Verification items for the finished model (mm, model axes). Face numbers are marked on the shaded views. A direction names the side the tool comes from. Round coordinates to 2 decimals unless told otherwise and drop trailing zeros. Loops run counter-clockwise (first coordinate to the right, second up) from the corner with the lowest first, then second, coordinate; pieces in that order, holes last. Notation, with made-up numbers: (61.25, 22) - (112.25, 22) arc R28 ccw to (112.25, 53) - close; hole circle Ø3 at (50, 74.5). An arc over 180 degrees is marked (long way). Use a Markdown table: item, result. Add a question column.
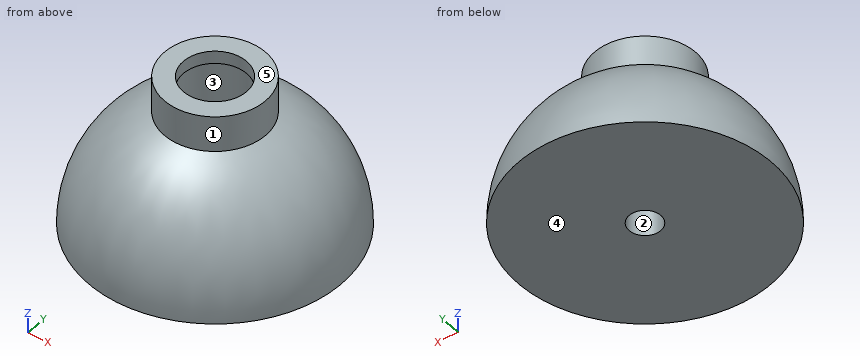
```python
from build123d import *

# Parameters (mm, degrees)
F1_R     = 25.4
F1_R_2   = 10.16
F2_DEPTH = 25.4
F3_R     = 25.39999
F4_DEPTH = 30.48
F7_D     = 16.51
F8_DEPTH = 7.62
F9_START = 27.94
F9_DEPTH = 2.54


# Not quite as in the source:
# - a variable given as a bare number and used for a length is read in inches; the dataset says mm whatever the document's units were
# - a fillet or chamfer is up to 0.001 mm smaller than in the source, because OpenCascade refuses the exact size


with BuildPart() as f2:
    # F1 (on Top) → F2 (new body)
    with BuildSketch(Plane.XY):
        Circle(F1_R)
        Circle(F1_R_2, mode=Mode.SUBTRACT)
        Circle(F1_R_2)
    extrude(amount=F2_DEPTH)

    # F3 (radius 25.4 in the source; OpenCascade refuses exactly that, so slightly less here)
    f3_edges = [f2.edges().sort_by_distance(p)[0] for p in [
        (-25.4, 0, 25.4),
    ]]
    fillet(f3_edges, radius=F3_R)

    # F1 (on Top) → F4 (join)
    with BuildSketch(Plane.XY):
        Circle(F1_R_2)
    extrude(amount=F4_DEPTH)

    # F7 (through all)
    with Locations(Plane(origin=(0, 0, 0), x_dir=(1, 0, 0), z_dir=(0, 0, -1))):
        with Locations((0, 0)):
            Hole(F7_D / 2)

    # F6 (on face) → F8 (join)
    with BuildSketch(Plane.XY):
        with BuildLine():
            ThreePointArc((-6.35, 0), (0, -6.35), (6.35, 0))
            Line((6.35, 0), (3.175, 0))
            ThreePointArc((3.175, 0), (0, -3.175), (-3.175, 0))
            Line((-3.175, 0), (-6.35, 0))
        make_face()
        with BuildLine():
            Line((3.175, 0), (6.35, 0))
            ThreePointArc((6.35, 0), (0, 6.35), (-6.35, 0))
            Line((-6.35, 0), (-3.175, 0))
            ThreePointArc((-3.175, 0), (0, 3.175), (3.175, 0))
        make_face()
        with BuildLine():
            Line((8.255, 0), (6.35, 0))
            ThreePointArc((6.35, 0), (0, -6.35), (-6.35, 0))
            Line((-6.35, 0), (-8.255, 0))
            ThreePointArc((-8.255, 0), (0, -8.255), (8.255, 0))
        make_face()
        with BuildLine():
            ThreePointArc((-6.35, 0), (0, 6.35), (6.35, 0))
            Line((6.35, 0), (8.255, 0))
            ThreePointArc((8.255, 0), (0, 8.255), (-8.255, 0))
            Line((-8.255, 0), (-6.35, 0))
        make_face()
    extrude(amount=F8_DEPTH)

    # F6 (on face) → F9 (join)
    with BuildSketch(Plane.XY.offset(F9_START)):
        with BuildLine():
            Line((8.255, 0), (6.35, 0))
            ThreePointArc((6.35, 0), (0, -6.35), (-6.35, 0))
            Line((-6.35, 0), (-8.255, 0))
            ThreePointArc((-8.255, 0), (0, -8.255), (8.255, 0))
        make_face()
        with BuildLine():
            ThreePointArc((-6.35, 0), (0, 6.35), (6.35, 0))
            Line((6.35, 0), (8.255, 0))
            ThreePointArc((8.255, 0), (0, 8.255), (-8.255, 0))
            Line((-8.255, 0), (-6.35, 0))
        make_face()
    extrude(amount=F9_DEPTH)


solid = f2.part
```
Q1. Release check for a two-part mould opening along Z. For the marked faces 3, 4 and 5 record: +Z half, -Z half, draft (parallel to the pull), parting line (faces both ways), or undercut.
Q2. Go/stop test with flat-tipped pins: pin 1 Ø10 at (x, z) = (-14, 23.5) entering from -Y; pin 2 Ø4 at (x, z) = (-1, 13) entering from +Y; pin 3 Ø4 at (x, z) = (-6.5, 7) entering from -Y. Record where each tip stops, or that it passes through.
Q3. Section check A-A on z = 25.5. Record the cut outline in (x, y) (3 decimals).
Q4. Set-up check for the marked faces 1 and 2: record each of +Z, -Z, +X, -X, +Y, -Y from which the full face is reachable in a straight line by a thin tool's end or side.
Q5. Thickness scan on line 1 along Y through (x, z) = (0, 28.95); line 2 along Z through (x, y) = (-7.5, 1.5); line 3 along Y through (x, z) = (0, 5) (3 decimals). Record the ranges inside material, lowest first.
Determined:
| question | item | result |
|---|---|---|
| 1 | face 3 | undercut |
| 1 | face 4 | -Z half |
| 1 | face 5 | +Z half |
| 2 | pin 1 | stops at y = -12.06 |
| 2 | pin 2 | stops at y = 22.88 |
| 2 | pin 3 | stops at y = -24.25 |
| 3 | outline | circle Ø20.32 at (0, 0); hole circle Ø16.51 at (0, 0) |
| 4 | face 1 | +Z |
| 4 | face 2 | +Z, -Z |
| 5 | line 1 | y = -10.16 to -6.35, 6.35 to 10.16 |
| 5 | line 2 | z = 0 to 7.62, 27.94 to 30.48 |
| 5 | line 3 | y = -24.903 to -3.175, 3.175 to 24.903 |
